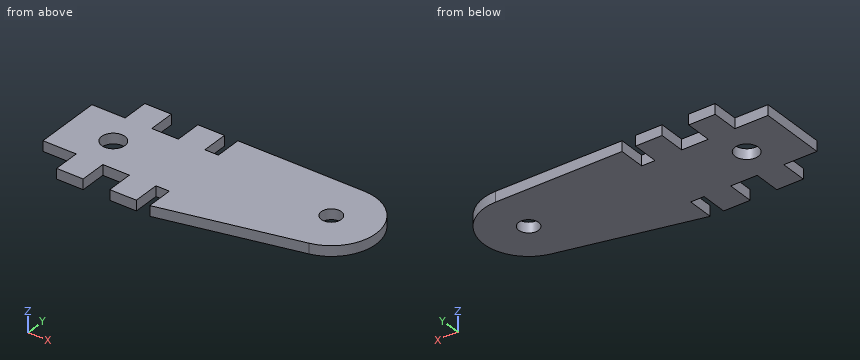
from build123d import *

# Parameters (mm, degrees)
SKETCH1_R           = 1.75
SKETCH1_R_2         = 1.5
BOSS_EXTRUDE1_DEPTH = 1.55


with BuildPart() as part:
    # Sketch1 → Boss-Extrude1 (new body)
    with BuildSketch(Plane.XY):
        with BuildLine():
            Line((5, 0), (9, 0))
            Line((9, 0), (9, 4))
            Line((9, 4), (13, 4))
            Line((13, 4), (13, 0))
            Line((13, 0), (17, 0))
            Line((17, 0), (17, 4))
            Line((17, 4), (19.021561934, 4))
            Line((19.021561934, 4), (19.021561934, 0))
            Line((19.021561934, 0), (39.557599026, 4.677766061))
            ThreePointArc((39.557599026, 4.677766061), (44.762590659, 12.008417985), (38.059495851, 17.999988357))
            Line((38.059495851, 17.999988357), (19.021561934, 17.999988357))
            Line((19.021561934, 17.999988357), (19.021561934, 13.999988357))
            Line((19.021561934, 13.999988357), (17, 13.999988357))
            Line((17, 13.999988357), (17, 17.999988357))
            Line((17, 17.999988357), (13, 17.999988357))
            Line((13, 17.999988357), (13, 13.999988357))
            Line((13, 13.999988357), (9, 13.999988357))
            Line((9, 13.999988357), (9, 17.999988357))
            Line((9, 17.999988357), (5, 17.999988357))
            Line((5, 17.999988357), (5, 13.999988357))
            Line((5, 13.999988357), (0, 13.999988357))
            Line((0, 13.999988357), (0, 4))
            Line((0, 4), (5, 4))
            Line((5, 4), (5, 0))
        make_face()
        with Locations(Location((6.9, 9, 0), (0, 0, 180))):
            Circle(SKETCH1_R, mode=Mode.SUBTRACT)
        with Locations(Location((38.059495851, 11.254645274, 0), (0, 0, 180))):
            Circle(SKETCH1_R_2, mode=Mode.SUBTRACT)
    extrude(amount=BOSS_EXTRUDE1_DEPTH)


solid = part.part
The model under review builds one solid part; all positions refer to its coordinate system, in mm. Round coordinates to 2 decimals unless told otherwise and drop trailing zeros. Loops run counter-clockwise (first coordinate to the right, second up) from the corner with the lowest first, then second, coordinate; pieces in that order, holes last. Notation, with made-up numbers: (-16.5, 37.25) -> (0.5, 37.25) arc R24 cw to (0.5, 73.25) -> close; hole circle Ø1 at (-3, 22). An arc over 180 degrees is marked (long way). Answer as CSV lines item,"result".
1) Add section C-C on z = 1.1. Write out the cut boundary in (x, y), plus the area to 3 significant figures.
Geometry results:
outline,"(0, 4) -> (5, 4) -> (5, 0) -> (9, 0) -> (9, 4) -> (13, 4) -> (13, 0) -> (17, 0) -> (17, 4) -> (19.02, 4) -> (19.02, 0) -> (39.56, 4.68) arc R6.75 ccw to (38.06, 18) -> (19.02, 18) -> (19.02, 14) -> (17, 14) -> (17, 18) -> (13, 18) -> (13, 14) -> (9, 14) -> (9, 18) -> (5, 18) -> (5, 14) -> (0, 14) -> close; hole circle Ø3.5 at (6.9, 9); hole circle Ø3 at (38.06, 11.25)"
area,"610 mm²"
2) For P1, Ø0.8, axis at x = 18, z = 0.5, coming from the +Y side; P2, Ø0.8, axis at y = 16.5, z = 1, coming from the -X side; P3, Ø0.5, axis at x = 11.5, z = 1, coming from the -Y side, all flat-tipped, find the tip position at first contact; note any pin that passes through.
Geometry results:
P1,"stops at y = 14"
P2,"stops at x = 5"
P3,"stops at y = 4"
3) Add section D-D on x = 18. Write out the cut boundary in (y, z), plus the area to 3 significant figures.
Geometry results:
outline,"(4, 0) -> (14, 0) -> (14, 1.55) -> (4, 1.55) -> close"
area,"15.5 mm²"
4) To check wall thickness, follow line 1 along X through (y, z) = (16, 0.75); line 2 along X through (y, z) = (17.25, 0.45); line 3 along Y through (x, z) = (6.9, 0.9). State the ranges of each line that lie inside material, in increasing order. Write a range as from..to.
Geometry results:
line 1,"x = 5..9, 13..17, 19.02..42.85"
line 2,"x = 5..9, 13..17, 19.02..41.15"
line 3,"y = 0..7.25, 10.75..18"
5) Add section A-A on x = 6.9. Write out the cut boundary in (y, z), plus the area to 3 significant figures.
Geometry results:
outline,"(0, 0) -> (7.25, 0) -> (7.25, 1.55) -> (0, 1.55) -> close; (10.75, 0) -> (18, 0) -> (18, 1.55) -> (10.75, 1.55) -> close"
area,"22.5 mm²"
6) Add section B-B on y = 9. Write out the cut boundary in (x, z), plus the area to 3 significant figures.
Geometry results:
outline,"(0, 0) -> (5.15, 0) -> (5.15, 1.55) -> (0, 1.55) -> close; (8.65, 0) -> (44.42, 0) -> (44.42, 1.55) -> (8.65, 1.55) -> close"
area,"63.4 mm²"
